CAD build for the part. Positions are in the model's coordinates, mm. A direction names the side the tool comes from. Coordinates: 2 decimals unless noted, no trailing zeros. Order: outer loops, then holes, each group sorted by start corner. A loop starts at its lowest first (then second) coordinate and runs counter-clockwise, first axis right, second up. Notation, with made-up numbers: (19, 40.5) - (42, 40.5) arc R10 cw to (42, 56.5) - close; hole circle Ø5 at (1.5, 63). An arc over 180 degrees is marked (long way). Return JSON: item names as keys, results as strings.
Autodesk Inventor part; units mm, degrees
ref_plane "Plano de trabajo3" through (0, 0, -60) normal (0, 0, 1) x (1, 0, 0)
ref_plane "YZ Plane" through (0, 0, 0) normal (1, 0, 0) x (0, 1, 0)
ref_plane "XZ Plane" through (0, 0, 0) normal (0, 1, 0) x (-1, 0, 0)
sketch "Boceto1" plane through (0, 0, 0) normal (0, 0, 1) x (1, 0, 0)
  line L0 (0, 124.4663) -> (0, -121.5162) construction
  line L1 (-141.4483, 0) -> (147.5578, 0) construction
  circle A0 centre (0, 0) radius 17.5
  dimension "d0" = 35
extrude "Extrusión1" add sketch "Boceto1" along normal blind 30
ref_plane "Plano de trabajo1" through (0, 0, -30) normal (0, 0, 1) x (1, 0, 0)
sketch "Boceto2" plane through (0, 0, -30) normal (0, 0, 1) x (1, 0, 0)
  circle A0 centre (0, 0) radius 42.5
  dimension "d4" = 85
loft "Solevación1" add profiles "Boceto2" section 2 edges at (-17.5, 0, 0)
ref_plane "Plano de trabajo2" through (0, 0, -55) normal (0, 0, 1) x (1, 0, 0)
sketch "Boceto3" plane through (0, 0, -55) normal (0, 0, 1) x (1, 0, 0)
  circle A0 centre (0, 0) radius 42.5
  dimension "d10" = 85
loft "Solevación2" add profiles "Boceto3" section 2 edges at (-42.5, 0, -30)
shell "Vaciado1" thickness 3 outward yes removed faces 2 at (-10.6049, 7.3037, -55) at (4.3663, -1.0762, 30)
sketch "Boceto4" plane through (0, 0, -55) normal (0, 0, -1) x (-1, 0, 0)
  circle A0 centre (0, 0) radius 44.5
  circle A1 centre (0, 0) radius 42.5
  line L0 (-2.5, 42.4264) -> (-2.5, 36.4244)
  line L1 (-2.5, 36.4244) -> (2.5, 36.4244)
  line L2 (2.5, 36.4244) -> (2.5, 42.4264)
  line L3 (-61.729, 0) -> (90.2911, 0) construction
  line L4 (0, 48.1461) -> (0, -48.1461) construction
  circle A2 centre (0, 0) radius 37 construction
  circle A3 centre (0, 0) radius 40 construction
  circle A4 centre (0, 0) radius 38.5 construction
  arc A5 (-2.5, 38.5) -> (2.5, 38.5) centre (0, 38.5) ccw
  line L5 (-35.4923, -23.3783) -> (-30.2945, -20.3773)
  arc A6 (-32.092, -21.4151) -> (-34.592, -17.0849) centre (-33.342, -19.25) ccw
  line L6 (-32.7945, -16.0472) -> (-37.9923, -19.0481)
  line L7 (37.9923, -19.0481) -> (32.7945, -16.0472)
  arc A7 (34.592, -17.0849) -> (32.092, -21.4151) centre (33.342, -19.25) ccw
  line L8 (30.2945, -20.3773) -> (35.4923, -23.3783)
  dimension "d21" = 77
  dimension "d16" = 85
  dimension "d17" = 74
  dimension "d18" = 80
  dimension "d19" = 5
  dimension "d20" = 6.002
  dimension "d22" = 5
  dimension "d25" = 360
extrude "Extrusión2" add sketch "Boceto4" against normal blind 3 contours L2 A5 L1 L0 A1 | A1 L8 A7 L7 | L6 A6 L5 A1 | A5 L1
ref_plane "Plano de trabajo3" through (0, 0, -60) normal (0, 0, 1) x (1, 0, 0)
sketch "Boceto5" plane through (0, 0, -60) normal (0, 0, 1) x (1, 0, 0)
  line L0 (0, 47.3974) -> (0, -47.5019) construction
  line L1 (54.9107, 0) -> (-68.9978, 0) construction
  circle A0 centre (0, 0) radius 38.5 construction
  circle A1 centre (0, 38.5) radius 2.5
  circle A2 centre (-33.342, -19.25) radius 2.5
  circle A3 centre (33.342, -19.25) radius 2.5
  dimension "d30" = 77
  dimension "d31" = 5
  dimension "d34" = 360
extrude "Extrusión3" add sketch "Boceto5" along normal blind 5
sketch "Boceto6" plane through (33.342, -19.25, -60) normal (0, 0, -1) x (-1, 0, 0)
  circle A0 centre (0, 0) radius 1.525
  circle A1 centre (0, 0) radius 2.5 construction
  circle A2 centre (66.684, 0) radius 1.525
  circle A3 centre (33.342, 57.75) radius 1.525
  point P0 (33.342, 19.25)
  dimension "d38" = 3.05
  dimension "d39" = 0.975
  dimension "d42" = 360
extrude "Extrusión4" cut sketch "Boceto6" against normal blind 5
properties part number "CAPSULA 1 MEDIDOR ESPORAS"
Item 1: Band-saw the part on A-A, the plane x = 0. List the corners of the cut face in (y, z) (3 decimals).
Findings below:
{"outline": "(-45.5, -55) - (-42.5, -55) - (-42.5, -30) - (-17.5, 0) - (-17.5, 30) - (-20.5, 30) - (-20.5, 1.086) - (-45.5, -28.914) - close; (17.5, 0) - (42.5, -30) - (42.5, -52) - (36, -52) - (36, -60) - (36.975, -60) - (36.975, -55) - (40.025, -55) - (40.025, -60) - (41, -60) - (41, -55) - (45.5, -55) - (45.5, -28.914) - (20.5, 1.086) - (20.5, 30) - (17.5, 30) - close"}
Item 2: Drop flat-ended pins along their axis: P1, Ø1, axis at x = 33.5, y = -12.5, coming from the -Z side; P2, Ø2.5, axis at x = -33.342, y = -19.25, coming from the +Z side; P3, Ø4, axis at x = -16, z = -7.5, coming from the -Y side; P4, Ø2.5, axis at x = -0.5, y = 38.5, coming from the -Z side. Give the stop position or say it passes through.
Findings below:
{"P1": "stops at z = -22.51", "P2": "stops at z = -19.01", "P3": "stops at y = -24.94", "P4": "stops at z = -60"}
Item 3: Band-saw the part on B-B, the plane z = -37.5. List the corners of the cut face in (x, y).
Findings below:
{"outline": "circle Ø91 at (0, 0); hole circle Ø85 at (0, 0)"}
Item 4: Mould opens along Y. For faces 1 (the flat face through (33, -21, -60)), 2 (the cylindrical face through (-31.205, -17.953, -53.521)), 3 (the conical face through (10.181, 19.574, -0.791)) say: released by +Y, released by -Y, zero draft, split by the parting line, or undercut.
Findings below:
{"face 1": "zero draft", "face 2": "undercut", "face 3": "split by the parting line"}
Item 5: Which spindle directions (+Z, -Z, +X, -X, +Y, -Y) get a long thin tool onto all of the face, cutting with end or side? Do faces 4 (the flat face through (1, 40, -60)), 5 (the flat face through (34, -20, -52)), 6 (the flat face through (-36.316, -18.08, -53.521)). Say none if no direction does.
Findings below:
{"face 4": "-Z, +X, -X, +Y, -Y", "face 5": "none", "face 6": "-Z"}
Item 6: Wall check: L1, parallel to X at y = -19, z = -56; L2, parallel to Y at x = 5, z = -7; L3, parallel to Y at x = 15.5, z = -45. Give the ranges that are in metal, low to high. Write a range as [from, to].
Findings below:
{"L1": "x = [-35.83, -34.85], [-31.84, -30.85], [30.85, 31.84], [34.85, 35.83]", "L2": "y = [-26.78, -22.79], [22.79, 26.78]", "L3": "y = [-42.78, -39.57], [39.57, 42.78]"}
Item 7: Band-saw the part on C-C, the plane z = 22.5. List the corners of the cut face in (x, y), then the cut area to 3 significant figures.
Findings below:
{"outline": "circle Ø41 at (0, 0); hole circle Ø35 at (0, 0)", "area": "358 mm²"}
